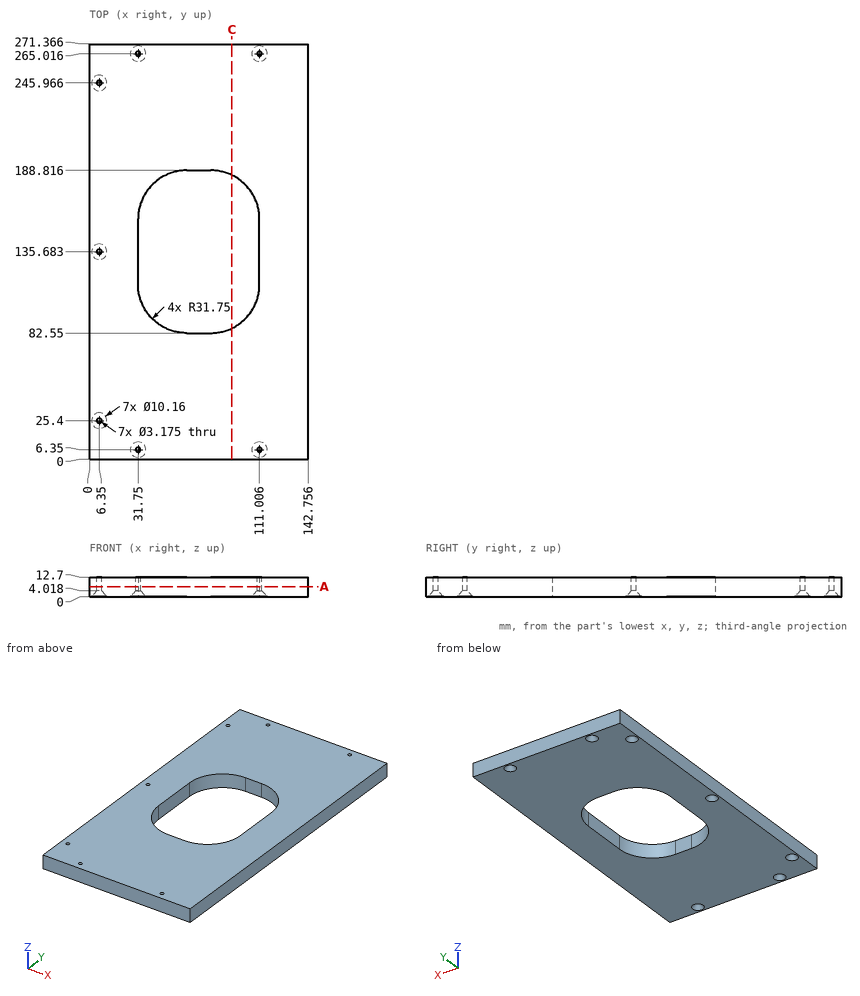
Study the drawing (mm; zero at the part's minimum x, y, z) and answer. Give positions to 0.01 mm unless a question says otherwise; leave off trailing zeros. Order: outer loops, then holes, each group sorted by start corner. A loop starts at its lowest first (then second) coordinate and runs counter-clockwise, first axis right, second up. Notation, with made-up numbers: (42, -39.5) - (98, -39.5) arc R18 cw to (98, -30.5) - close; hole circle Ø5 at (88.25, 89.5). An arc over 180 degrees is marked (long way). Answer as CSV lines item,"result". Start each with the question number.
Q1. Find the intervals of material crossed by L1, parallel to Y at x = 6.35, z = 11 (1 decimal); L2, parallel to X at y = 6.35, z = 10 (1 decimal); L3, parallel to X at y = 25.4, z = 10.25 (1 decimal), in increasing order. Write a range as [from, to].
Q2. The part is cut by section A-A (z = 6.75). Give the number of separate pieces and of enclosed holes in the cut face, then the cut area to 3 significant figures.
Q3. The part is cut by section C-C (x = 93). Write down the section's boundary in (y, z) (1 decimal), then the cut area to 3 significant figures.
Q4. Given pin 1 Ø2.5 at (x, y) = (6.35, 245.97) entering from +Z; pin 2 Ø4 at (x, y) = (6.35, 135.68) entering from -Z, each flat-ended and moving along its own axis, determine where each tip first touches the part or whether it passes through.
Check result:
1,L1,"y = [0, 23.8], [27, 134.1], [137.3, 244.4], [247.6, 271.4]"
1,L2,"x = [0, 30.2], [33.3, 109.4], [112.6, 142.8]"
1,L3,"x = [0, 4.8], [7.9, 142.8]"
2,separate pieces,"1"
2,enclosed holes,"8"
2,area,"31,100 mm²"
3,outline,"(0, 0) - (85.7, 0) - (85.7, 12.7) - (0, 12.7) - close; (185.7, 0) - (271.4, 0) - (271.4, 12.7) - (185.7, 12.7) - close"
3,area,"2,180 mm²"
4,pin 1,"passes through"
4,pin 2,"stops at z = 3.54"
